```python
from build123d import *

# Parameters (mm, degrees)
F1_DEPTH = 2
F2_R     = 0.99999
F3_R     = 2
F6_DEPTH = 3


# Not quite as in the source:
# - a fillet or chamfer is up to 0.001 mm smaller than in the source, because OpenCascade refuses the exact size


with BuildPart() as f1:
    # F0 (on Top) → F1 (new body)
    with BuildSketch(Plane.XY):
        with BuildLine():
            Line((73.5948921635, -24.4738152558), (30.4890723007, 20.4280804346))
            ThreePointArc((30.4890723007, 20.4280804346), (0, 36.7), (-30.4890723007, 20.4280804346))
            Line((-30.4890723007, 20.4280804346), (-71.107024482, -18.5651536595))
            ThreePointArc((-71.107024482, -18.5651536595), (-88.6093292458, -48.364956076), (-73.5948921635, -79.4925254511))
            Line((-73.5948921635, -79.4925254511), (-30.4890723007, -124.3944211415))
            ThreePointArc((-30.4890723007, -124.3944211415), (0, -140.666340707), (30.4890723007, -124.3944211415))
            Line((30.4890723007, -124.3944211415), (71.107024482, -85.4011870475))
            ThreePointArc((71.107024482, -85.4011870475), (88.6093292458, -55.601384631), (73.5948921635, -24.4738152558))
        make_face()
        with BuildLine():
            Line((-28.1743255129, -124.7318742155), (-6.0285815603, -109.2252573607))
            ThreePointArc((-6.0285815603, -109.2252573607), (-3.6939889059, -111.0624273724), (-0.85, -111.9210562896))
            Line((-0.85, -111.9210562896), (-0.85, -138.9560177561))
            ThreePointArc((-0.85, -138.9560177561), (-16.1612014632, -135.0117198682), (-28.1743255129, -124.7318742155))
        make_face(mode=Mode.SUBTRACT)
        with BuildLine():
            ThreePointArc((-59.9226587205, -50.3870367891), (-59.1807775846, -53.2636891654), (-57.4403870983, -55.6712932586))
            Line((-57.4403870983, -55.6712932586), (-73.8376241337, -77.1659381522))
            ThreePointArc((-73.8376241337, -77.1659381522), (-83.618782922, -64.7434058486), (-86.9351098111, -49.2840283695))
            Line((-86.9351098111, -49.2840283695), (-59.9226587205, -50.3870367891))
        make_face(mode=Mode.SUBTRACT)
        with BuildLine():
            ThreePointArc((-5, -3.3166247904), (0, 6), (5, -3.3166247904))
            Line((5, -3.3166247904), (5, -6.2449979984))
            ThreePointArc((5, -6.2449979984), (7.847410611, -1.555039132), (7.0036615021, 3.8663581784))
            Line((7.0036615021, 3.8663581784), (29.1494054547, 19.3729750332))
            Line((29.1494054547, 19.3729750332), (72.4860077697, -25.7693190449))
            Line((72.4860077697, -25.7693190449), (56.0887707343, -47.2639639384))
            ThreePointArc((56.0887707343, -47.2639639384), (50.7063118949, -46.1997279693), (45.9040856171, -48.8534205162))
            Line((45.9040856171, -48.8534205162), (48.830020546, -48.9728961925))
            ThreePointArc((48.830020546, -48.9728961925), (57.9348912774, -54.3488450807), (48.4220272071, -58.9645697978))
            Line((48.4220272071, -58.9645697978), (45.4960922782, -58.8450941215))
            ThreePointArc((45.4960922782, -58.8450941215), (50.0659736435, -61.8814810638), (55.5172812862, -61.2596238927))
            Line((55.5172812862, -61.2596238927), (70.1074551181, -84.0195880634))
            Line((70.1074551181, -84.0195880634), (29.1494054547, -123.3393157402))
            Line((29.1494054547, -123.3393157402), (7.0036615021, -107.8326988854))
            ThreePointArc((7.0036615021, -107.8326988854), (7.847410611, -102.411301575), (5, -97.7213427086))
            Line((5, -97.7213427086), (5, -100.6497159166))
            ThreePointArc((5, -100.6497159166), (0, -109.966340707), (-5, -100.6497159166))
            Line((-5, -100.6497159166), (-5, -97.7213427086))
            ThreePointArc((-5, -97.7213427086), (-7.847410611, -102.411301575), (-7.0036615021, -107.8326988854))
            Line((-7.0036615021, -107.8326988854), (-29.1494054547, -123.3393157402))
            Line((-29.1494054547, -123.3393157402), (-72.4860077697, -78.1970216621))
            Line((-72.4860077697, -78.1970216621), (-56.0887707343, -56.7023767685))
            ThreePointArc((-56.0887707343, -56.7023767685), (-50.7063118949, -57.7666127376), (-45.9040856171, -55.1129201908))
            Line((-45.9040856171, -55.1129201908), (-48.830020546, -54.9934445145))
            ThreePointArc((-48.830020546, -54.9934445145), (-57.9348912774, -49.6174956263), (-48.4220272071, -45.0017709092))
            Line((-48.4220272071, -45.0017709092), (-45.4960922782, -45.1212465855))
            ThreePointArc((-45.4960922782, -45.1212465855), (-50.0659736435, -42.0848596432), (-55.5172812862, -42.7067168143))
            Line((-55.5172812862, -42.7067168143), (-70.1074551181, -19.9467526436))
            Line((-70.1074551181, -19.9467526436), (-29.1494054547, 19.3729750332))
            Line((-29.1494054547, 19.3729750332), (-7.0036615021, 3.8663581784))
            ThreePointArc((-7.0036615021, 3.8663581784), (-7.847410611, -1.555039132), (-5, -6.2449979984))
            Line((-5, -6.2449979984), (-5, -3.3166247904))
        make_face(mode=Mode.SUBTRACT)
        with BuildLine():
            Line((0.85, -138.9560177561), (0.85, -111.9210562896))
            ThreePointArc((0.85, -111.9210562896), (3.6939889059, -111.0624273724), (6.0285815603, -109.2252573607))
            Line((6.0285815603, -109.2252573607), (28.1743255129, -124.7318742155))
            ThreePointArc((28.1743255129, -124.7318742155), (16.1612014632, -135.0117198682), (0.85, -138.9560177561))
        make_face(mode=Mode.SUBTRACT)
        with BuildLine():
            ThreePointArc((56.9484628744, -60.3421712992), (58.8793530111, -58.0844778314), (59.8532998529, -55.2778884308))
            Line((59.8532998529, -55.2778884308), (86.8657509435, -56.3808968503))
            ThreePointArc((86.8657509435, -56.3808968503), (82.300050413, -71.5184248765), (71.5386367063, -83.1021354698))
            Line((71.5386367063, -83.1021354698), (56.9484628744, -60.3421712992))
        make_face(mode=Mode.SUBTRACT)
        with BuildLine():
            ThreePointArc((-56.9484628744, -43.6241694078), (-58.8793530111, -45.8818628756), (-59.8532998529, -48.6884522762))
            Line((-59.8532998529, -48.6884522762), (-86.8657509435, -47.5854438566))
            ThreePointArc((-86.8657509435, -47.5854438566), (-82.300050413, -32.4479158305), (-71.5386367063, -20.8642052372))
            Line((-71.5386367063, -20.8642052372), (-56.9484628744, -43.6241694078))
        make_face(mode=Mode.SUBTRACT)
        with BuildLine():
            ThreePointArc((-0.85, 7.9547155826), (-3.6939889059, 7.0960866654), (-6.0285815603, 5.2589166537))
            Line((-6.0285815603, 5.2589166537), (-28.1743255129, 20.7655335085))
            ThreePointArc((-28.1743255129, 20.7655335085), (-16.1612014632, 31.0453791612), (-0.85, 34.9896770491))
            Line((-0.85, 34.9896770491), (-0.85, 7.9547155826))
        make_face(mode=Mode.SUBTRACT)
        with BuildLine():
            ThreePointArc((59.9226587205, -53.5793039179), (59.1807775846, -50.7026515416), (57.4403870983, -48.2950474484))
            Line((57.4403870983, -48.2950474484), (73.8376241337, -26.8004025548))
            ThreePointArc((73.8376241337, -26.8004025548), (83.618782922, -39.2229348584), (86.9351098111, -54.6823123374))
            Line((86.9351098111, -54.6823123374), (59.9226587205, -53.5793039179))
        make_face(mode=Mode.SUBTRACT)
        with BuildLine():
            ThreePointArc((0.85, 34.9896770491), (16.1612014632, 31.0453791612), (28.1743255129, 20.7655335085))
            Line((28.1743255129, 20.7655335085), (6.0285815603, 5.2589166537))
            ThreePointArc((6.0285815603, 5.2589166537), (3.6939889059, 7.0960866654), (0.85, 7.9547155826))
            Line((0.85, 7.9547155826), (0.85, 34.9896770491))
        make_face(mode=Mode.SUBTRACT)
    extrude(amount=F1_DEPTH)

    # F2 (radius 1 in the source; OpenCascade refuses exactly that, so slightly less here)
    f2_edges = [f1.edges().sort_by_distance(p)[0] for p in [
        (-5, -3.316625, 1),
        (-5, -6.244998, 1),
        (5, -3.316625, 1),
        (5, -6.244998, 1),
        (48.830021, -48.972896, 1),
        (45.904086, -48.853421, 1),
        (48.422027, -58.96457, 1),
        (45.496092, -58.845094, 1),
        (5, -100.649716, 1),
        (5, -97.721343, 1),
        (-5, -97.721343, 1),
        (-5, -100.649716, 1),
        (-48.830021, -54.993445, 1),
        (-45.904086, -55.11292, 1),
        (-48.422027, -45.001771, 1),
        (-45.496092, -45.121247, 1),
    ]]
    fillet(f2_edges, radius=F2_R)

    # F3
    f3_edges = [f1.edges().sort_by_distance(p)[0] for p in [
        (6.028582, 5.258917, 1),
        (0.85, 7.954716, 1),
        (7.003662, 3.866358, 1),
        (-0.85, 7.954716, 1),
        (-7.003662, 3.866358, 1),
        (-6.028582, 5.258917, 1),
        (28.174326, 20.765534, 1),
        (-28.174326, 20.765534, 1),
        (-0.85, 34.989677, 1),
        (0.85, 34.989677, 1),
    ]]
    fillet(f3_edges, radius=F3_R)

    # F5 (on face) → F6 (join)
    with BuildSketch(Plane.XY.offset(2)):
        with BuildLine():
            ThreePointArc((-49.0618129875, -55.126955847), (-57.9348912774, -49.6174956263), (-48.6421626961, -44.8498058529))
            ThreePointArc((-48.6421626961, -44.8498058529), (-47.2571276636, -44.5640122932), (-47.5429212234, -43.1789772607))
            ThreePointArc((-47.5429212234, -43.1789772607), (-59.9332259985, -49.5358969586), (-48.1024549453, -56.8818439194))
            ThreePointArc((-48.1024549453, -56.8818439194), (-47.7046899302, -55.5247208621), (-49.0618129875, -55.126955847))
        make_face()
        with BuildLine():
            ThreePointArc((-6.8571428571, -99.8457106779), (0, -111.966340707), (6.8571428571, -99.8457106779))
            ThreePointArc((6.8571428571, -99.8457106779), (5.4849212464, -99.5036465744), (5.1428571429, -100.8758681852))
            ThreePointArc((5.1428571429, -100.8758681852), (0, -109.966340707), (-5.1428571429, -100.8758681852))
            ThreePointArc((-5.1428571429, -100.8758681852), (-5.4849212464, -99.5036465744), (-6.8571428571, -99.8457106779))
        make_face()
        with BuildLine():
            ThreePointArc((49.0618129875, -48.83938486), (57.9348912774, -54.3488450807), (48.6421626961, -59.1165348541))
            ThreePointArc((48.6421626961, -59.1165348541), (47.2571276636, -59.4023284138), (47.5429212234, -60.7873634463))
            ThreePointArc((47.5429212234, -60.7873634463), (59.9332259985, -54.4304437484), (48.1024549453, -47.0844967876))
            ThreePointArc((48.1024549453, -47.0844967876), (47.7046899302, -48.4416198449), (49.0618129875, -48.83938486))
        make_face()
        with BuildLine():
            ThreePointArc((-5.1428571429, -3.0904725218), (0, 6), (5.1428571429, -3.0904725218))
            ThreePointArc((5.1428571429, -3.0904725218), (5.4849212464, -4.4626941326), (6.8571428571, -4.1206300291))
            ThreePointArc((6.8571428571, -4.1206300291), (0, 8), (-6.8571428571, -4.1206300291))
            ThreePointArc((-6.8571428571, -4.1206300291), (-5.4849212464, -4.4626941326), (-5.1428571429, -3.0904725218))
        make_face()
    extrude(amount=F6_DEPTH)


solid = f1.part
```
CAD build for the part. Positions are in the model's coordinates, mm. A direction names the side the tool comes from. Round coordinates to 2 decimals unless told otherwise and drop trailing zeros. Loops run counter-clockwise (first coordinate to the right, second up) from the corner with the lowest first, then second, coordinate; pieces in that order, holes last. Notation, with made-up numbers: (71.25, 81.25) - (130.25, 81.25) arc R17 ccw to (130.25, 97.25) - close; hole circle Ø10 at (10.5, 16). An arc over 180 degrees is marked (long way). Return JSON: item names as keys, results as strings. Group by question number.
Q1. Tool access for faces 4 (the face through (-0.504, -140.663, 0.986)), 5 (the face through (16.359, -134.908, 0.986)): list every direction of +Z, -Z, +X, -X, +Y, -Y with a clear straight run to the whole face (end or side of a thin tool).
Q2. Flat gauge pins, fed straight in: pin 1 Ø0.6 at (y, z) = (26.5, 1) entering from -X; pin 2 Ø1.6 at (y, z) = (25.5, 1) entering from +X; pin 3 Ø14 at (x, y) = (0, -103.97) entering from -Z; pin 4 Ø1.5 at (x, z) = (-2, 1.5) entering from +Y. Where does each tip first touch, or does it go through?
Q3. Band-saw the part on B-B on z = 4.25. Give the cut face in (x, y), plus the area to 3 significant figures.
Q4. Band-saw the part on C-C on x = -35.5. Give the cut face in (y, z).
Q5. Two-plate mould, pull along Y, no slides. Class faces 1 (the face through (-88.585, -47.862, 0.986)), 2 (the face through (-50.514, 1.204, 0.986)), 3 (the face through (-64.35, -32.08, 0.99)): +Y half, -Y half, draft (parallel to the pull), parting line (faces both ways), or undercut.
Q6. Drill centre lines: line 1 along X through (y, z) = (0, 4.05); line 2 along X through (y, z) = (-83, 1.7); line 3 along X through (y, z) = (0, 1.15). Where is each one in solid material? Low to high. Write a range as [from, to].
Q7. Band-saw the part on A-A on x = 19. Give the cut face in (y, z), plus the area to 3 significant figures.
Solutions:
{
 "1": {"face 4": "+Z, -Z, -Y", "face 5": "+Z, -Z"},
 "2": {"pin 1": "stops at x = -25.7", "pin 2": "stops at x = 27.14", "pin 3": "stops at z = 0", "pin 4": "stops at y = 36.68"},
 "3": {"outline": "(-49.06, -55.13) arc R6 cw (long way) to (-48.64, -44.85) arc R1 ccw to (-47.54, -43.18) arc R8 ccw (long way) to (-48.1, -56.88) arc R1 ccw to start; (-6.86, -99.85) arc R8 ccw (long way) to (6.86, -99.85) arc R1 ccw to (5.14, -100.88) arc R6 cw (long way) to (-5.14, -100.88) arc R1 ccw to start; (-6.86, -4.12) arc R1 ccw to (-5.14, -3.09) arc R6 cw (long way) to (5.14, -3.09) arc R1 ccw to (6.86, -4.12) arc R8 ccw (long way) to start; (47.54, -60.79) arc R8 ccw (long way) to (48.1, -47.08) arc R1 ccw to (49.06, -48.84) arc R6 cw (long way) to (48.64, -59.12) arc R1 ccw to start", "area": "249 mm^2"},
 "4": {"outline": "(-119.17, 0) - (-116.72, 0) - (-116.72, 2) - (-119.17, 2) - close; (13.28, 0) - (15.62, 0) - (15.62, 2) - (13.28, 2) - close"},
 "5": {"face 1": "parting line", "face 2": "+Y half", "face 3": "undercut"},
 "6": {"line 1": "x = [-8, -6], [6, 8]", "line 2": "x = [-70.23, -67.88], [69.45, 71.47], [71.69, 74.57]", "line 3": "x = [-51.77, -49.33], [-8, -6], [6, 8], [47.75, 50.1]"},
 "7": {"outline": "(-135.37, 0) - (-133.36, 0) - (-133.36, 2) - (-135.37, 2) - close; (-118.31, 0) - (-116.23, 0) - (-116.23, 2) - (-118.31, 2) - close; (12.27, 0) - (14.34, 0) - (14.34, 2) - (12.27, 2) - close; (29.39, 0) - (31.4, 0) - (31.4, 2) - (29.39, 2) - close", "area": "16.3 mm^2"}
}
